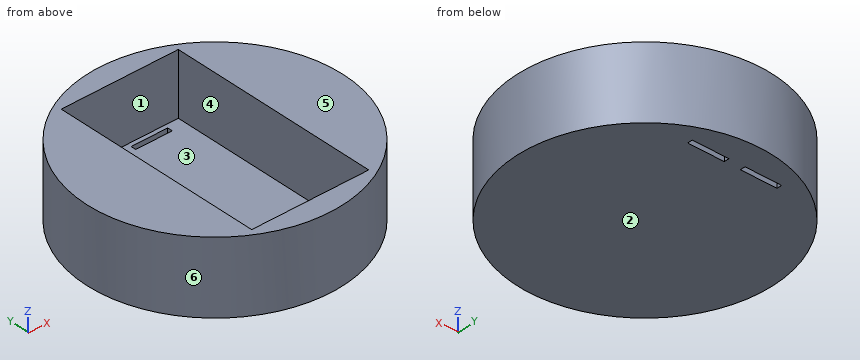
from build123d import *

# Parameters (mm, degrees)
F0_R     = 35
F1_DEPTH = 20
F2_W     = 32
F2_H     = 58
F3_DEPTH = 17
F4_W     = 10
F4_H     = 1.4
F5_DEPTH = 5
F6_W     = 10
F6_H     = 1.4
F7_DEPTH = 5


with BuildPart() as f1:
    # F0 (on Top) → F1 (new body)
    with BuildSketch(Plane.XY):
        Circle(F0_R)
    extrude(amount=F1_DEPTH)

    # F2 (on face) → F3 (cut)
    with BuildSketch(Plane.XY.offset(20)):
        Rectangle(F2_W, F2_H)
    extrude(amount=-F3_DEPTH, mode=Mode.SUBTRACT)

    # F4 (on face) → F5 (cut)
    with BuildSketch(Plane.XY.offset(3)):
        with Locations((-7.300642, 27.198469)):
            Rectangle(F4_W, F4_H)
    extrude(amount=-F5_DEPTH, mode=Mode.SUBTRACT)

    # F6 (on Top) → F7 (cut)
    with BuildSketch(Plane.XY):
        with Locations((7.077963, 27.159134)):
            Rectangle(F6_W, F6_H)
    extrude(amount=F7_DEPTH, mode=Mode.SUBTRACT)


solid = f1.part
Geometry: final body of the model. Coordinates: model frame, mm. Face numbers are marked on the shaded views. A direction names the side the tool comes from. Coordinates: 2 decimals unless noted, no trailing zeros. Write each loop counter-clockwise with the first axis right and the second up, starting at its lowest first coordinate (ties: lowest second). Pieces come first, ordered by that corner, then holes. Notation, with made-up numbers: (84, 3) - (108, 3) arc R34 ccw to (108, 41) - close; hole circle Ø11 at (-34, 76.5). An arc over 180 degrees is marked (long way). Return JSON: item names as keys, results as strings.
Item 1: Section query C-C (x = 0). Output: boundary loops of the cut face in (y, z), and give its area (3 significant figures).
Completed:
{"outline": "(-35, 0) - (35, 0) - (35, 20) - (29, 20) - (29, 3) - (-29, 3) - (-29, 20) - (-35, 20) - close", "area": "414 mm2"}
Item 2: Line query: L1, parallel to Y at x = 0, z = 6; L2, parallel to X at y = 19, z = 12.5; L3, parallel to Z at x = 1.5, y = 12.5. Output: solid intervals per line, ascending.
Completed:
{"L1": "y = -35 to -29, 29 to 35", "L2": "x = -29.39 to -16, 16 to 29.39", "L3": "z = 0 to 3"}
Item 3: Section query B-B (z = 15.5). Output: boundary loops of the cut face in (x, y).
Completed:
{"outline": "circle Ø70 at (0, 0); hole (-16, -29) - (16, -29) - (16, 29) - (-16, 29) - close"}
Item 4: Section query A-A (y = 0). Output: boundary loops of the cut face in (x, z).
Completed:
{"outline": "(-35, 0) - (35, 0) - (35, 20) - (16, 20) - (16, 3) - (-16, 3) - (-16, 20) - (-35, 20) - close"}
Item 5: Pull-direction query (X, two-part tool) for the marked faces 3, 4, 5 and 6; classes: +X half, -X half, draft (parallel to the pull), parting line (faces both ways), or undercut.
Completed:
{"face 3": "undercut", "face 4": "undercut", "face 5": "draft", "face 6": "parting line"}
Item 6: Reachability of the marked faces 1 and 2 from +Z, -Z, +X, -X, +Y, -Y: full face, straight path, thin tool, end or side. Return the list, or none.
Completed:
{"face 1": "+Z", "face 2": "-Z, +X, -X, +Y, -Y"}
Item 7: Pin query (flat end, axial travel): pin 1 Ø2 at (x, z) = (-3, 4.5) entering from -Y; pin 2 Ø1.5 at (x, z) = (-7.5, 1.5) entering from -Y; pin 3 Ø1 at (x, z) = (0, 8.5) entering from +Y. Return the tip coordinate at first contact, or that it passes through.
Completed:
{"pin 1": "stops at y = -34.94", "pin 2": "stops at y = -34.34", "pin 3": "stops at y = 35"}
